Source: three-view drawing plus pictorial views. Frame: mm from the lowest corner of the part. A direction names the side the tool comes from. Round coordinates to 2 decimals unless told otherwise and drop trailing zeros. Loops run counter-clockwise (first coordinate to the right, second up) from the corner with the lowest first, then second, coordinate; pieces in that order, holes last. Notation, with made-up numbers: (51, 66.25) -> (97, 66.25) arc R21 ccw to (97, 98.25) -> close; hole circle Ø9 at (23.5, 38). An arc over 180 degrees is marked (long way). Return JSON: item names as keys, results as strings. Group by question number.
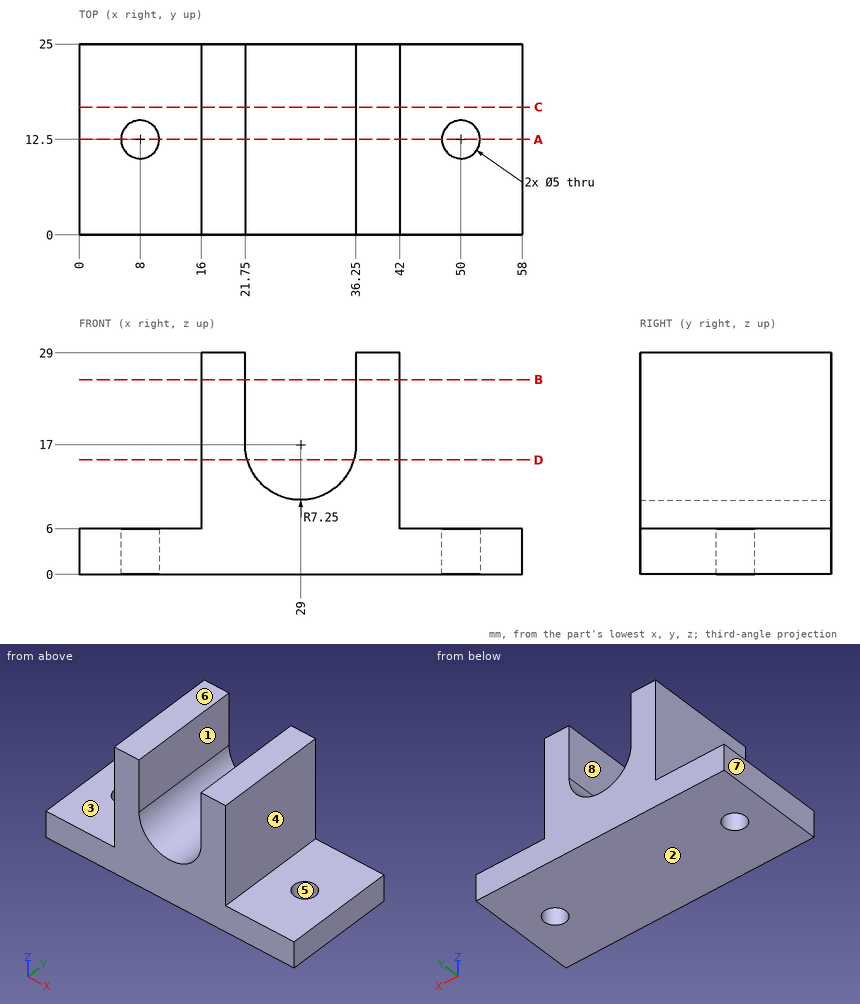
(1) Ray query, line 1 (X direction, y = 2.75, z = 22.5); line 2 (Z direction, x = 7.5, y = 6.5); line 3 (X direction, y = 15.25, z = 7). Return the intervals inside material, ascending.
(2) Pin query (flat end, axial travel): pin 1 (10 mm diameter, centred on x = 30, y = 18, fed in from +Z); pin 2 (5 mm diameter, centred on x = 4.5, y = 13.5, fed in from +Z); pin 3 (7 mm diameter, centred on y = 6.5, z = 22, fed in from -X). Return the tip coordinate at first contact, or that it passes through.
(3) Cut plane A-A (y = 12.5). Return loops of the section in (x, z).
(4) Mould query, pull axis X, two halves, no side actions, for the marked faces 5, 6, 7 and 8. Classes: released by +X, released by -X, zero draft, split by the parting line, or undercut.
(5) Cut plane C-C (y = 16.75). Return loops of the section in (x, z).
(6) Cut plane D-D (z = 15). Return loops of the section in (x, y).
(7) Set-up query: the marked faces 1, 2, 3 and 4. Return all of +Z, -Z, +X, -X, +Y, -Y with unobstructed straight access to the full face (end or side cutting, diameter ignored); none if empty.
(8) Cut plane B-B (z = 25.5). Return loops of the section in (x, y), and give its area (4 significant figures).
Answers follow:
{
 "1": {"line 1": "16 to 21.75, 36.25 to 42", "line 2": "0 to 6", "line 3": "16 to 42"},
 "2": {"pin 1": "z = 12.93", "pin 2": "z = 6", "pin 3": "x = 16"},
 "3": {"outline": "(0, 0) -> (5.5, 0) -> (5.5, 6) -> (0, 6) -> close; (10.5, 0) -> (47.5, 0) -> (47.5, 6) -> (42, 6) -> (42, 29) -> (36.25, 29) -> (36.25, 17) arc R7.25 cw to (21.75, 17) -> (21.75, 29) -> (16, 29) -> (16, 6) -> (10.5, 6) -> close; (52.5, 0) -> (58, 0) -> (58, 6) -> (52.5, 6) -> close"},
 "4": {"face 5": "undercut", "face 6": "zero draft", "face 7": "released by -X", "face 8": "undercut"},
 "5": {"outline": "(0, 0) -> (58, 0) -> (58, 6) -> (42, 6) -> (42, 29) -> (36.25, 29) -> (36.25, 17) arc R7.25 cw to (21.75, 17) -> (21.75, 29) -> (16, 29) -> (16, 6) -> (0, 6) -> close"},
 "6": {"outline": "(16, 0) -> (22.03, 0) -> (22.03, 25) -> (16, 25) -> close; (35.97, 0) -> (42, 0) -> (42, 25) -> (35.97, 25) -> close"},
 "7": {"face 1": "+Z, +Y, -Y", "face 2": "-Z, +X, -X, +Y, -Y", "face 3": "+Z, -X, +Y, -Y", "face 4": "+Z, +X, +Y, -Y"},
 "8": {"outline": "(16, 0) -> (21.75, 0) -> (21.75, 25) -> (16, 25) -> close; (36.25, 0) -> (42, 0) -> (42, 25) -> (36.25, 25) -> close", "area": "287.5 mm^2"}
}
